from build123d import *

# Parameters (mm, degrees)
SKETCH_2_R          = 6
SKETCH_2_R_2        = 3
EXTRUDE_1_DEPTH     = 19
SKETCH_3_R          = 5
SKETCH_3_R_2        = 3.5
CUT_EXTRUDE_1_DEPTH = 0.5
CUT_EXTRUDE_START   = -0.5
SKETCH_4_R          = 5
SKETCH_4_R_2        = 3.5
CUT_EXTRUDE_2_DEPTH = 0.5
FILLET_1_R          = 0.4


with BuildPart() as part:
    # 草图2 → 凸台-拉伸1 (new body)
    with BuildSketch(Plane.XY):
        Circle(SKETCH_2_R)
        Circle(SKETCH_2_R_2, mode=Mode.SUBTRACT)
    extrude(amount=EXTRUDE_1_DEPTH)

    # 草图3 → 切除-拉伸1 (cut)
    with BuildSketch(Plane.XY.offset(19)):
        Circle(SKETCH_3_R)
        Circle(SKETCH_3_R_2, mode=Mode.SUBTRACT)
    extrude(amount=-CUT_EXTRUDE_1_DEPTH, mode=Mode.SUBTRACT)

    # 草图4 → 切除-拉伸2 (cut)
    with BuildSketch(Plane(origin=(0, 0, 0), x_dir=(-1, 0, 0), z_dir=(0, 0, -1)).offset(CUT_EXTRUDE_START)):
        with Locations(Location((0, 0, 0), (0, 0, 180))):
            Circle(SKETCH_4_R)
        with Locations(Location((0, 0, 0), (0, 0, 180))):
            Circle(SKETCH_4_R_2, mode=Mode.SUBTRACT)
    extrude(amount=CUT_EXTRUDE_2_DEPTH, mode=Mode.SUBTRACT)

    # 圆角1
    fillet_1_edges = [part.edges().sort_by_distance(p)[0] for p in [
        (-5, 0, 19),
        (-6, 0, 0),
        (-5, 0, 0),
        (-6, 0, 19),
    ]]
    fillet(fillet_1_edges, radius=FILLET_1_R)


solid = part.part
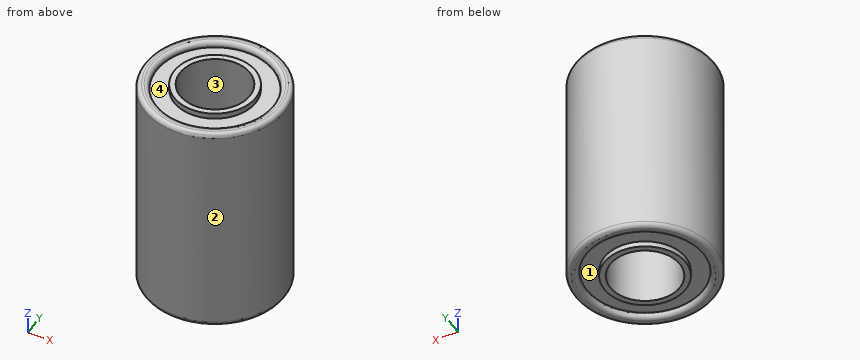
The model under review builds one solid part; all positions refer to its coordinate system, in mm. Face numbers are marked on the shaded views. A direction names the side the tool comes from. Round coordinates to 2 decimals unless told otherwise and drop trailing zeros. Loops run counter-clockwise (first coordinate to the right, second up) from the corner with the lowest first, then second, coordinate; pieces in that order, holes last. Notation, with made-up numbers: (20, 5.25) -> (78, 5.25) arc R19 ccw to (78, 34.25) -> close; hole circle Ø7 at (-15.75, -9.5). An arc over 180 degrees is marked (long way). Return JSON: item names as keys, results as strings.
(1) For line 1 (Y direction, x = 0, z = 7.25); line 2 (Y direction, x = 1.25, z = 12.75); line 3 (Z direction, x = 3.5, y = 3), list the stretches that pass through material, from the lowest coordinate up.
Solved:
{"line 1": "-6 to -3, 3 to 6", "line 2": "-5.87 to -2.73, 2.73 to 5.87", "line 3": "0.5 to 18.5"}
(2) For pin 1 (2 mm diameter, centred on x = 4, z = 7, fed in from +Y); pin 2 (1.5 mm diameter, centred on x = 1.5, z = 10, fed in from -Y); pin 3 (5 mm diameter, centred on x = -2.5, y = 0.5, fed in from -Z); pin 4 (1 mm diameter, centred on y = 2.5, z = 4, fed in from -X), all flat-tipped, find the tip position at first contact; note any pin that passes through.
Solved:
{"pin 1": "y = 5.2", "pin 2": "y = -5.95", "pin 3": "z = 0", "pin 4": "x = -5.66"}
(3) For the marked faces 3 and 4, list the 3-axis set-ups (+Z, -Z, +X, -X, +Y, -Y) from which the entire face can be reached by the end or side of a thin tool; tool diameter is ignored.
Solved:
{"face 3": "+Z, -Z", "face 4": "+Z"}
(4) The part is to be moulded in two halves that separate along X. For the marked faces 1 and 2, say which applies: released by +X, released by -X, zero draft, split by the parting line, or undercut.
Solved:
{"face 1": "undercut", "face 2": "split by the parting line"}
(5) Add section C-C on z = 8.75. Write out the cut boundary in (x, y), plus the area to 3 significant figures.
Solved:
{"outline": "circle Ø12 at (0, 0); hole circle Ø6 at (0, 0)", "area": "84.8 mm2"}
